Part model, mm, in its own coordinate system. A direction names the side the tool comes from. Coordinates: 2 decimals unless noted, no trailing zeros. Loops run counter-clockwise (first coordinate to the right, second up) from the corner with the lowest first, then second, coordinate; pieces in that order, holes last. Notation, with made-up numbers: M 29,40 L 86,40 A24 cw 86,66 Z; hole C -29.5,-25.5 d6. An arc over 180 degrees is marked long. Use a Markdown table: item, result. Add a question column.
1) Wall check: probe 1 along X at (y, z) = (65.5, 0.4); probe 2 along Y at (x, z) = (62.5, 5.7); probe 3 along Y at (x, z) = (129, 1.5). Give the ranges that are in metal, low to high. Write a range as from..to.
2) Tool access for faces 5 (the flat face through (121, 15, 3)), 6 (the flat face through (114, 63, 3)), 7 (the flat face through (247, 40, 3)), 8 (the flat face through (-3, 20, 3)), 9 (the flat face through (75, 66, 3)): list every direction of +Z, -Z, +X, -X, +Y, -Y with a clear straight run to the whole face (end or side of a thin tool).
3) Band-saw the part on A-A (y = 35.5). List the corners of the cut face in (x, z).
4) Band-saw the part on B-B (x = 138). List the corners of the cut face in (y, z).
5) Pull direction Y, two halves, no side cores. Call faces 1 (the flat face through (164, 77, 3)), 2 (the flat face through (244, 65, 3)), 3 (the flat face through (121, 45, 3)), 4 (the flat face through (247, 20, 3)): released by +Y, released by -Y, zero draft, split by the parting line, or undercut.
6) Band-saw the part on D-D (y = 75). List the corners of the cut face in (x, z), plus the area to 3 significant figures.
7) Pin check, flat tips, straight feed: pin 1 Ø3 at (x, z) = (149.5, 3.5) entering from +Y; pin 2 Ø1.8 at (y, z) = (74.5, 3.5) entering from +X; pin 3 Ø1.8 at (y, z) = (64.5, 2) entering from -X; pin 4 Ø3 at (x, z) = (101.5, 2.5) entering from -Y. Stop position of each tip, or through.
from build123d import *

# Parameters (mm, degrees)
SKETCH_1_W      = 204
SKETCH_1_H      = 30
EXTRUDE_1_DEPTH = 6
FILLET_2_R      = 6


with BuildPart() as part:
    # Эскиз1 → Бобышка-Вытянуть1 (new body)
    with BuildSketch(Plane.XY):
        Polygon((0, 20), (0, 0), (244, 0), (244, 20), (250, 20), (250, 40), (244, 40), (244, 90), (220, 90), (220, 93), (161, 93), (161, 87), (164, 87), (164, 66), (134, 66), (134, 60), (114, 60), (114, 66), (34, 66), (34, 60), (14, 60), (14, 66), (0, 66), (0, 40), (-6, 40), (-6, 20), align=None)
        with Locations((122, 30)):
            Rectangle(SKETCH_1_W, SKETCH_1_H, mode=Mode.SUBTRACT)
    extrude(amount=EXTRUDE_1_DEPTH)

    # Скругление2
    fillet_2_edges = [part.edges().sort_by_distance(p)[0] for p in [
        (161, 93, 3),
    ]]
    fillet(fillet_2_edges, radius=FILLET_2_R - 0.0001)  # a hair under: the kernel refuses the full size


solid = part.part
Entries:
| question | item | result |
|---|---|---|
| 1 | probe 1 | 0..14, 34..114, 134..244 |
| 1 | probe 2 | 0..15, 45..66 |
| 1 | probe 3 | 0..15, 45..60 |
| 2 | face 5 | +Z, -Z |
| 2 | face 6 | +Z, -Z, +Y |
| 2 | face 7 | +Z, -Z, +X, +Y |
| 2 | face 8 | +Z, -Z, -X, -Y |
| 2 | face 9 | +Z, -Z, -X, +Y |
| 3 | outline | M -6,0 L 20,0 L 20,6 L -6,6 Z; M 224,0 L 250,0 L 250,6 L 224,6 Z |
| 4 | outline | M 0,0 L 15,0 L 15,6 L 0,6 Z; M 45,0 L 66,0 L 66,6 L 45,6 Z |
| 5 | face 1 | undercut |
| 5 | face 2 | zero draft |
| 5 | face 3 | undercut |
| 5 | face 4 | released by -Y |
| 6 | outline | M 164,0 L 244,0 L 244,6 L 164,6 Z |
| 6 | area | 480 mm2 |
| 7 | pin 1 | y = 66 |
| 7 | pin 2 | x = 244 |
| 7 | pin 3 | x = 0 |
| 7 | pin 4 | y = 0 |
